from build123d import *

# Parameters (mm, degrees)
F0_W     = 12
F0_H     = 2.5
F1_DEPTH = 30
F3_D     = 4.1
F5_D     = 4.1
F5_DEPTH = 2.501
F0_R     = 4.2799
F6_DEPTH = 13


with BuildPart() as f1:
    # F0 (on Top) → F1 (new body)
    with BuildSketch(Plane.XY):
        with Locations((-23.0367250374, -16.25)):
            Rectangle(F0_W, F0_H)
        with Locations((18.9632749626, -16.25)):
            Rectangle(F0_W, F0_H)
        with BuildLine():
            ThreePointArc((-12.1578164158, 1.5), (12.25, 0), (-12.1578164158, -1.5))
            Line((-12.1578164158, -1.5), (-29.0367250374, -1.5))
            Line((-29.0367250374, -1.5), (-29.0367250374, -4))
            Line((-29.0367250374, -4), (-17.0367250374, -4))
            Line((-17.0367250374, -4), (-17.0367250374, -15))
            Line((-17.0367250374, -15), (-17.0367250374, -17.5))
            Line((-17.0367250374, -17.5), (12.9632749626, -17.5))
            Line((12.9632749626, -17.5), (12.9632749626, -15))
            Line((12.9632749626, -15), (12.9632749626, -11.7559985643))
            ThreePointArc((12.9632749626, -11.7559985643), (15.1017388634, 8.8423686477), (-3.9079399616, 17.0580774197))
            ThreePointArc((-3.9079399616, 17.0580774197), (-12.340911411, 12.4077357139), (-17.0367250374, 4))
            Line((-17.0367250374, 4), (-29.0367250374, 4))
            Line((-29.0367250374, 4), (-29.0367250374, 1.5))
            Line((-29.0367250374, 1.5), (-12.1578164158, 1.5))
        make_face()
    extrude(amount=F1_DEPTH)

    # F3 (through all)
    with Locations(Plane(origin=(0, 4, 0), x_dir=(-1, 0, 0), z_dir=(0, 1, 0))):
        with Locations((23.0367250374, 7.5), (23.0367250374, 22.5)):
            Hole(F3_D / 2)

    # F5 (through all, one way)
    with BuildSketch(Plane(origin=(0, -15, 0), x_dir=(-1, 0, 0), z_dir=(0, 1, 0))):
        with Locations((-18.9632749626, 22.5), (-18.9632749626, 7.5)):
            Circle(F5_D / 2)
    extrude(amount=-F5_DEPTH, mode=Mode.SUBTRACT)

    # F0 (on Top) → F6 (join)
    with BuildSketch(Plane.XY):
        with BuildLine():
            Line((25.4464586396, 23.7830572941), (-3.9079399616, 17.0580774197))
            ThreePointArc((-3.9079399616, 17.0580774197), (15.1017388634, 8.8423686477), (12.9632749626, -11.7559985643))
            Line((12.9632749626, -11.7559985643), (33.8875290885, 7.9880305701))
            ThreePointArc((33.8875290885, 7.9880305701), (19.3342866208, 10.3636090033), (25.4464586396, 23.7830572941))
        make_face()
        with BuildLine():
            ThreePointArc((36.7986610424, 14.7375), (33.3017440504, 21.9951615751), (25.4464586396, 23.7830572941))
            ThreePointArc((25.4464586396, 23.7830572941), (19.3342866208, 10.3636090033), (33.8875290885, 7.9880305701))
            ThreePointArc((33.8875290885, 7.9880305701), (36.0398547105, 11.062243994), (36.7986610424, 14.7375))
        make_face()
        with Locations((27.5187610424, 14.7375)):
            Circle(F0_R, mode=Mode.SUBTRACT)
    extrude(amount=F6_DEPTH)


solid = f1.part
The model under review builds one solid part; all positions refer to its coordinate system, in mm. A direction names the side the tool comes from. Give positions to 0.01 mm unless a question says otherwise; leave off trailing zeros. Order: outer loops, then holes, each group sorted by start corner. A loop starts at its lowest first (then second) coordinate and runs counter-clockwise, first axis right, second up. Notation, with made-up numbers: M -11.5,39.5 L 2.5,39.5 A6 ccw 2.5,50.5 Z; hole C 30,45 d11. An arc over 180 degrees is marked long. Answer in a Markdown table with one row per item. Add a question column.
1. Add section C-C on z = 22.5. Count the separate pieces of the cut face and the enclosed holes in it, plus the area to 3 significant figures.
2. Add section D-D on z = 18.75. State the section outline as (x, y) points, plus the area to 3 significant figures.
3. To check wall thickness, follow line 1 along Z through (x, y) = (16, 12); line 2 along X through (y, z) = (-14.5, 14.5); line 3 along X through (y, z) = (-15.5, 11.25). State the ranges of each line that lie inside material, in increasing order.
4. Machinability: for faces 4 (the flat face through (12.963, -13, 15)), 5 (the cylindrical face through (21.01, -16.23, 22.59)), 6 (the flat face through (-23, -4, 15)), which of the approach directions +Z, -Z, +X, -X, +Y, -Y give a long, thin tool a straight path to every point of the face, cutting with its end or side? Answer none if there is none.
5. For pin 1 Ø1 at (y, z) = (0.5, 24) entering from -X; pin 2 Ø12 at (y, z) = (-4, 14.5) entering from +X; pin 3 Ø3 at (y, z) = (-16.5, 18) entering from +X; pin 4 Ø3 at (x, y) = (10.5, 18.5) entering from -Z, all flat-tipped, find the tip position at first contact; note any pin that passes through.
6. Mouldability with a two-part tool opening along X and no side actions: class faces 1 (the flat face through (24.963, -16, 15)), 2 (the flat face through (-29.037, -16, 15)), 3 (the cylindrical face through (-23.48, 2.73, 5.5)) as released by +X, released by -X, zero draft, split by the parting line, or undercut.
7. Add section A-A on x = -18. State the section outline as (y, z) points.
8. Add section B-B on y = 2.5. State the section outline as (x, z) points, plus the area to 3 significant figures.
The answers:
| question | item | result |
|---|---|---|
| 1 | separate pieces | 5 |
| 1 | enclosed holes | 0 |
| 1 | area | 635 mm2 |
| 2 | outline | M -29.04,-17.5 L 24.96,-17.5 L 24.96,-15 L 12.96,-15 L 12.96,-11.76 A17.5 ccw long -17.04,4 L -29.04,4 L -29.04,1.5 L -12.16,1.5 A12.25 cw long -12.16,-1.5 L -29.04,-1.5 L -29.04,-4 L -17.04,-4 L -17.04,-15 L -29.04,-15 Z |
| 2 | area | 676 mm2 |
| 3 | line 1 | 0 to 13 |
| 3 | line 2 | -17.04 to 12.96 |
| 3 | line 3 | -29.04 to 24.96 |
| 4 | face 4 | +Z, -Z, +X |
| 4 | face 5 | -Y |
| 4 | face 6 | +Z, -Z, -X |
| 5 | pin 1 | x = 12.21 |
| 5 | pin 2 | x = 27.34 |
| 5 | pin 3 | x = 24.96 |
| 5 | pin 4 | z = 0 |
| 6 | face 1 | released by +X |
| 6 | face 2 | released by -X |
| 6 | face 3 | undercut |
| 7 | outline | M -17.5,0 L -15,0 L -15,30 L -17.5,30 Z; M -4,0 L -1.5,0 L -1.5,30 L -4,30 Z; M 1.5,0 L 4,0 L 4,30 L 1.5,30 Z |
| 8 | outline | M -29.04,0 L -11.99,0 L -11.99,30 L -29.04,30 Z; M 11.99,0 L 28.07,0 L 28.07,13 L 17.32,13 L 17.32,30 L 11.99,30 Z; hole C -23.04,7.5 d4.1; hole C -23.04,22.5 d4.1 |
| 8 | area | 785 mm2 |
